Could you check a few things on this model? Use its own coordinates, in mm. A direction names the side the tool comes from. Coordinates: 2 decimals unless noted, no trailing zeros. Loops run counter-clockwise (first coordinate to the right, second up) from the corner with the lowest first, then second, coordinate; pieces in that order, holes last.
from build123d import *

# Parameters (mm, degrees)
SKETCH3_W           = 100
SKETCH3_H           = 80
BOSS_EXTRUDE1_DEPTH = 3.18
SKETCH4_W           = 50.18
SKETCH4_H           = 3.18
CUT_EXTRUDE1_DEPTH  = 3.18
SKETCH5_W           = 3.18
SKETCH5_H           = 40.18
CUT_EXTRUDE2_DEPTH  = 3.18
SKETCH6_W           = 3.18
SKETCH6_H           = 19.91
CUT_EXTRUDE3_DEPTH  = 3.18


with BuildPart() as part:
    # Sketch3 → Boss-Extrude1 (new body)
    with BuildSketch(Plane.XY):
        Rectangle(SKETCH3_W, SKETCH3_H)
    extrude(amount=BOSS_EXTRUDE1_DEPTH)

    # Sketch4 → Cut-Extrude1 (cut)
    with BuildSketch(Plane.XY.offset(3.18)):
        with Locations((0, 38.41)):
            Rectangle(SKETCH4_W, SKETCH4_H)
    cut_extrude1 = extrude(amount=-CUT_EXTRUDE1_DEPTH, mode=Mode.SUBTRACT)

    # Mirror1: Cut-Extrude1 across plane
    add(cut_extrude1.mirror(Plane.ZX), mode=Mode.SUBTRACT)

    # Sketch5 → Cut-Extrude2 (cut)
    with BuildSketch(Plane.XY.offset(3.18)):
        with Locations((48.41, 0)):
            Rectangle(SKETCH5_W, SKETCH5_H)
    extrude(amount=-CUT_EXTRUDE2_DEPTH, mode=Mode.SUBTRACT)

    # Sketch6 → Cut-Extrude3 (cut)
    with BuildSketch(Plane.XY.offset(3.18)):
        with Locations((-48.41, 30.045)):
            Rectangle(SKETCH6_W, SKETCH6_H)
    cut_extrude3 = extrude(amount=-CUT_EXTRUDE3_DEPTH, mode=Mode.SUBTRACT)

    # Mirror2: Cut-Extrude3 across plane
    add(cut_extrude3.mirror(Plane.ZX), mode=Mode.SUBTRACT)


solid = part.part
(1) Imagine slicing it at B-B, the plane y = -3.5. Write out the boundary of the cut face in (x, z).
Answers:
outline: (-50, 0) - (46.82, 0) - (46.82, 3.18) - (-50, 3.18) - close
(2) For pin 1 (1 mm diameter, centred on y = -32, z = 1.5, fed in from -X); pin 2 (1 mm diameter, centred on x = 3.5, z = 2, fed in from -Y); pin 3 (4 mm diameter, centred on x = -6, y = -1, fed in from -Z); pin 4 (1.5 mm diameter, centred on x = 9.5, z = 1, fed in from +Y), each with a flat end and sliding along its axis, tell me the tip position at first contact or that it passes through.
Answers:
pin 1: stops at x = -46.82
pin 2: stops at y = -36.82
pin 3: stops at z = 0
pin 4: stops at y = 36.82
(3) Imagine slicing it at A-A, the plane z = 1.15. Write out the boundary of the cut face in (x, y), and give its area (3 significant figures).
Answers:
outline: (-50, -20.09) - (-46.82, -20.09) - (-46.82, -40) - (-25.09, -40) - (-25.09, -36.82) - (25.09, -36.82) - (25.09, -40) - (50, -40) - (50, -20.09) - (46.82, -20.09) - (46.82, 20.09) - (50, 20.09) - (50, 40) - (25.09, 40) - (25.09, 36.82) - (-25.09, 36.82) - (-25.09, 40) - (-46.82, 40) - (-46.82, 20.09) - (-50, 20.09) - close
area: 7,430 mm2
(4) Which directions (+Z, -Z, +X, -X, +Y, -Y) give clear straight access to the entire face, cutting with the end or side of a thin tool? Please do faces 5 (the face through (-46.82, 30, 2)), 6 (the face through (-48, -20.09, 2)), 7 (the face through (48, -20.09, 2)), 8 (the face through (25.09, 38, 2)), 9 (the face through (0, -36.82, 2)).
Answers:
face 5: +Z, -Z, -X, +Y
face 6: +Z, -Z, -X, -Y
face 7: +Z, -Z, +X
face 8: +Z, -Z, +Y
face 9: +Z, -Z, -Y
(5) We'd pull the mould along X, two halves only. Please class faces 1 (the face through (37, 40, 2)), 2 (the face through (-25.09, -38, 2)), 3 (the face through (50, -30, 2)), 4 (the face through (-25.09, 38, 2)): +X half, -X half, draft (parallel to the pull), parting line (faces both ways), or undercut.
Answers:
face 1: draft
face 2: undercut
face 3: +X half
face 4: undercut
(6) Imagine slicing it at C-C, the plane x = 23. Write out the boundary of the cut face in (y, z), and give its area (3 significant figures).
Answers:
outline: (-36.82, 0) - (36.82, 0) - (36.82, 3.18) - (-36.82, 3.18) - close
area: 234 mm2
(7) I need wall thicknesses on probe 1 along Y at (x, z) = (-17, 0.8); probe 2 along X at (y, z) = (20.5, 0.6); probe 3 along X at (y, z) = (-8, 0.35). Which ranges of each line are inside material? Lowest first, please.
Answers:
probe 1: y = -36.82 to 36.82
probe 2: x = -46.82 to 50
probe 3: x = -50 to 46.82
